Geometry check sheet. Reference: the model listing, model coordinates, mm. A direction names the side the tool comes from. Round coordinates to 2 decimals unless told otherwise and drop trailing zeros. Loops run counter-clockwise (first coordinate to the right, second up) from the corner with the lowest first, then second, coordinate; pieces in that order, holes last. Notation, with made-up numbers: (26, 76.25) - (42, 76.25) arc R9 cw to (42, 84.25) - close; hole circle Ø6 at (42, 73). An arc over 180 degrees is marked (long way). Answer in a Markdown table with one row per item. Add a question column.
```python
from build123d import *

# Parameters (mm, degrees)
SKETCH1_W           = 40
SKETCH1_H           = 40
SKETCH1_R           = 2.15
BOSS_EXTRUDE1_DEPTH = 20
FILLET1_R           = 5


with BuildPart() as part:
    # Sketch1 → Boss-Extrude1 (new body)
    with BuildSketch(Plane(origin=(0, 0, 0), x_dir=(1, 0, 0), z_dir=(0, 1, 0))):
        Rectangle(SKETCH1_W, SKETCH1_H)
        with Locations(Location((16, 16, 0), (0, 0, 270))):
            Circle(SKETCH1_R, mode=Mode.SUBTRACT)
        with Locations(Location((16, -16, 0), (0, 0, 270))):
            Circle(SKETCH1_R, mode=Mode.SUBTRACT)
        with Locations(Location((-16, -16, 0), (0, 0, 270))):
            Circle(SKETCH1_R, mode=Mode.SUBTRACT)
        with Locations(Location((-16, 16, 0), (0, 0, 270))):
            Circle(SKETCH1_R, mode=Mode.SUBTRACT)
        with BuildLine():
            Line((-5.5, 19), (5.5, 19))
            ThreePointArc((5.5, 19), (13.986600731, 13.986600731), (19, 5.5))
            Line((19, 5.5), (19, -5.5))
            ThreePointArc((19, -5.5), (13.986600731, -13.986600731), (5.5, -19))
            Line((5.5, -19), (-5.5, -19))
            ThreePointArc((-5.5, -19), (-13.986600731, -13.986600731), (-19, -5.5))
            Line((-19, -5.5), (-19, 5.5))
            ThreePointArc((-19, 5.5), (-13.986600731, 13.986600731), (-5.5, 19))
        make_face(mode=Mode.SUBTRACT)
    extrude(amount=BOSS_EXTRUDE1_DEPTH)

    # Fillet1
    fillet1_edges = [part.edges().sort_by_distance(p)[0] for p in [
        (20, 10, 20),
        (-20, 10, 20),
        (-20, 10, -20),
        (20, 10, -20),
    ]]
    fillet(fillet1_edges, radius=FILLET1_R)


solid = part.part
```
Q1. Cross-section at D-D, the plane z = -16. Enter the section's corners in (x, y).
Q2. Cross-section at C-C, the plane x = 0. Enter the section's corners in (y, z).
Q3. Scan lines: line 1 (X direction, y = 6.5, z = 4); line 2 (X direction, y = 4, z = 15); line 3 (X direction, y = 7.75, z = 16). Record each from-to range of solid material in increasing order. Write a range as from..to.
Q4. Depth check by flat-ended pin: P1, Ø3.5, axis at x = 16, z = -16, coming from the +Y side. Enter the tip coordinate at first touch or a pass-through.
Q5. Cross-section at B-B, the plane y = 1.5. Enter the section's corners in (x, z).
Q6. Release check for a two-part mould opening along X. For faces 1 (the flat face through (20, 10, 0)), 2 (the cylindrical face through (14.09, 9.86, -15.01)), 3 (the cylindrical face through (-19, 10, 18)) record: +X half, -X half, draft (parallel to the pull), parting line (faces both ways), or undercut.
Q7. Cross-section at A-A, the plane z = 2.5. Enter the section's corners in (x, y).
Q8. Set-up check for faces 4 (the flat face through (0, 10, -19)), 5 (the cylindrical face through (18, 10, 19)): record each of +Z, -Z, +X, -X, +Y, -Y from which the full face is reachable in a straight line by a thin tool's end or side.
Check sheet entries:
| question | item | result |
|---|---|---|
| 1 | outline | (-19.9, 0) - (-18.15, 0) - (-18.15, 20) - (-19.9, 20) - close; (-13.85, 0) - (-11.63, 0) - (-11.63, 20) - (-13.85, 20) - close; (11.63, 0) - (13.85, 0) - (13.85, 20) - (11.63, 20) - close; (18.15, 0) - (19.9, 0) - (19.9, 20) - (18.15, 20) - close |
| 2 | outline | (0, -20) - (20, -20) - (20, -19) - (0, -19) - close; (0, 19) - (20, 19) - (20, 20) - (0, 20) - close |
| 3 | line 1 | -20..-19, 19..20 |
| 3 | line 2 | -20..-17.9, -14.1..-12.89, 12.89..14.1, 17.9..20 |
| 3 | line 3 | -19.9..-18.15, -13.85..-11.63, 11.63..13.85, 18.15..19.9 |
| 4 | P1 | through |
| 5 | outline | (-20, -15) arc R5 ccw to (-15, -20) - (15, -20) arc R5 ccw to (20, -15) - (20, 15) arc R5 ccw to (15, 20) - (-15, 20) arc R5 ccw to (-20, 15) - close; hole (-19, -5.5) arc R19.78 ccw to (-5.5, -19) - (5.5, -19) arc R19.78 ccw to (19, -5.5) - (19, 5.5) arc R19.78 ccw to (5.5, 19) - (-5.5, 19) arc R19.78 ccw to (-19, 5.5) - close; hole circle Ø4.3 at (-16, -16); hole circle Ø4.3 at (-16, 16); hole circle Ø4.3 at (16, -16); hole circle Ø4.3 at (16, 16) |
| 6 | face 1 | +X half |
| 6 | face 2 | undercut |
| 6 | face 3 | -X half |
| 7 | outline | (-20, 0) - (-19, 0) - (-19, 20) - (-20, 20) - close; (19, 0) - (20, 0) - (20, 20) - (19, 20) - close |
| 8 | face 4 | +Y, -Y |
| 8 | face 5 | +Z, +X, +Y, -Y |
